Could you check a few things on this model? Use its own coordinates, in mm. A direction names the side the tool comes from. Give positions to 0.01 mm unless a question says otherwise; leave off trailing zeros. Order: outer loops, then holes, each group sorted by start corner. A loop starts at its lowest first (then second) coordinate and runs counter-clockwise, first axis right, second up. Notation, with made-up numbers: M -1,2.25 L 43,2.25 A25 ccw 43,27.25 Z; hole C 73.5,34.5 d11. An arc over 180 degrees is marked long. Use a Markdown table: item, result. Add a question column.
Item 1: For faces 1 (the face through (4.092, 1.732, -9.494)), 2 (the face through (3.9, 3.19, -9.47)), 3 (the face through (4.887, 0.253, -8.443)), which set-ups out of +Z, -Z, +X, -X, +Y, -Y let a thin tool reach every point of the face, with its end or its side?
Item 2: Suppose I cut it at A-A on x = 0. Count the separate pieces of the cut face and the enclosed holes in it, plus the area to 4 significant figures.
Item 3: Suppose I cut it at B-B on y = 1.25. Write out the boundary of the cut face in (x, z), plus the area to 3 significant figures.
Item 4: If I drill on L1, parallel to X at y = 1.9, z = 6; L2, parallel to Z at x = -10.5, y = 1; L3, parallel to X at y = 1.35, z = -5, over which ranges is the centre line in solid material (lowest first)? Write a range as from..to.
Item 5: If we mould it in two halves opening along Z, with no side actions, what happens to faces 4 (the face through (3.91, 0.31, -9.44)), 5 (the face through (-7.98, 1.73, 12.7)), 6 (the face through (7.691, 0.254, -9.901))? For each: released by +Z, released by -Z, zero draft, split by the parting line, or undercut.
Item 6: I'm going to push flat-ended pins straight in: pin 1 Ø3.5 at (x, z) = (10.39, 6) entering from +Y; pin 2 Ø2 at (x, y) = (2, 2) entering from +Z. Where does each tip first touch, or does it pass through?
from build123d import *

# Parameters (mm, degrees)
SKETCH_1_R          = 15
SKETCH_1_R_2        = 1.6
SKETCH_1_R_3        = 1.5
SKETCH_1_R_4        = 7
EXTRUDE_1_DEPTH     = 3.5
CUT_EXTRUDE_1_DEPTH = 8
FILLET_1_R          = 1
FILLET_2_R          = 1
CHAMFER_1_SIZE      = 0.5


with BuildPart() as part:
    # 草图1 → 凸台-拉伸1 (new body)
    with BuildSketch(Plane(origin=(0, 0, 0), x_dir=(1, 0, 0), z_dir=(0, 1, 0))):
        with Locations(Location((0, 0, 0), (0, 0, 270))):
            Circle(SKETCH_1_R)
        with Locations(Location((0, 12, 0), (0, 0, 270))):
            Circle(SKETCH_1_R_2, mode=Mode.SUBTRACT)
        with Locations(Location((10.392304845, -6, 0), (0, 0, 270))):
            Circle(SKETCH_1_R_2, mode=Mode.SUBTRACT)
        with Locations(Location((-10.392304845, -6, 0), (0, 0, 270))):
            Circle(SKETCH_1_R_2, mode=Mode.SUBTRACT)
        with Locations(Location((10.392304845, 6, 0), (0, 0, 270))):
            Circle(SKETCH_1_R_3, mode=Mode.SUBTRACT)
        with Locations(Location((0, -12, 0), (0, 0, 270))):
            Circle(SKETCH_1_R_3, mode=Mode.SUBTRACT)
        with Locations(Location((-10.392304845, 6, 0), (0, 0, 270))):
            Circle(SKETCH_1_R_3, mode=Mode.SUBTRACT)
        with Locations(Location((0, 0, 0), (0, 0, 270))):
            Circle(SKETCH_1_R_4, mode=Mode.SUBTRACT)
    extrude(amount=EXTRUDE_1_DEPTH)

    # 草图2 → 切除-拉伸1 (cut)
    with BuildSketch(Plane(origin=(0, 3.5, 0), x_dir=(1, 0, 0), z_dir=(0, 1, 0))):
        Polygon((3.690349309, 9.391530065), (6.310792277, 7.930955296), (9.125758213, 12.981335358), (6.505315246, 14.441910127), align=None)
    extrude(amount=-CUT_EXTRUDE_1_DEPTH, mode=Mode.SUBTRACT)

    # 圆角1
    fillet_1_edges = [part.edges().sort_by_distance(p)[0] for p in [
        (8.700707091, 1.75, -12.218743639),
        (6.095052455, 1.75, -13.705850414),
    ]]
    fillet(fillet_1_edges, radius=FILLET_1_R)

    # 圆角2
    fillet_2_edges = [part.edges().sort_by_distance(p)[0] for p in [
        (6.310792277, 1.75, -7.930955296),
        (3.690349309, 1.75, -9.391530065),
    ]]
    fillet(fillet_2_edges, radius=FILLET_2_R)

    # 倒角1
    chamfer_1_edges = [part.edges().sort_by_distance(p)[0] for p in [
        (10.392304845, 0, 4.4),
        (10.392304845, 3.5, 4.4),
        (-10.392304845, 0, 4.4),
        (-10.392304845, 3.5, 4.4),
        (0, 3.5, -7),
        (0, 0, 10.5),
        (0, 3.5, 10.5),
        (-10.392304845, 0, -7.5),
        (-10.392304845, 3.5, -7.5),
        (0, 0, -13.6),
        (0, 3.5, -13.6),
        (-7.446160806, 3.5, 13.021316725),
        (-7.446160806, 0, 13.021316725),
        (4.859185687, 3.5, -11.488560036),
        (5.603157458, 3.5, -13.552361106),
        (8.827728967, 3.5, -11.700311046),
        (4.859185687, 0, -11.488560036),
        (5.603157458, 0, -13.552361106),
        (8.827728967, 0, -11.700311046),
        (7.466276221, 3.5, -10.004029432),
        (7.466276221, 0, -10.004029432),
        (5.000570793, 3.5, -8.661242681),
        (5.000570793, 0, -8.661242681),
        (6.1975531, 3.5, -8.329389436),
        (6.1975531, 0, -8.329389436),
        (4.08878345, 3.5, -9.504769242),
        (4.08878345, 0, -9.504769242),
        (10.392304845, 0, -7.5),
        (10.392304845, 3.5, -7.5),
    ]]
    chamfer(chamfer_1_edges, length=CHAMFER_1_SIZE)


solid = part.part
Findings below:
| question | item | result |
|---|---|---|
| 1 | face 1 | +Y, -Y |
| 1 | face 2 | +Y |
| 1 | face 3 | -Y |
| 2 | separate pieces | 4 |
| 2 | enclosed holes | 0 |
| 2 | area | 32.55 mm^2 |
| 3 | outline | M 4.18,-10.27 A1 cw 4.56,-8.9 L 5.44,-8.42 A1 cw 6.8,-8.8 L 8.13,-11.2 A1 ccw 9.65,-11.48 A15 ccw long 5,-14.14 A1 ccw 5.54,-12.71 Z; hole C -10.39,6 d3.2; hole C -10.39,-6 d3; hole C 0,0 d14; hole C 0,-12 d3.2; hole C 0,12 d3; hole C 10.39,6 d3.2; hole C 10.39,-6 d3 |
| 3 | area | 492 mm^2 |
| 4 | L1 | x = -13.75..-11.99, -8.79..-3.61, 3.61..8.79, 11.99..13.75 |
| 4 | L2 | z = -10.71..-7.5, -4.5..4.4, 7.6..10.71 |
| 4 | L3 | x = -14.14..-11.51, -9.27..-4.9, 4.9..9.27, 11.51..14.14 |
| 5 | face 4 | undercut |
| 5 | face 5 | split by the parting line |
| 5 | face 6 | released by -Z |
| 6 | pin 1 | stops at y = 3.15 |
| 6 | pin 2 | stops at z = 14.97 |
